Check sheet for the modelled part. Datum: model origin and axes. Units: mm. Face numbers are marked on the shaded views. A direction names the side the tool comes from. Give positions to 0.01 mm unless a question says otherwise; leave off trailing zeros. Loops run counter-clockwise (first coordinate to the right, second up) from the corner with the lowest first, then second, coordinate; pieces in that order, holes last.
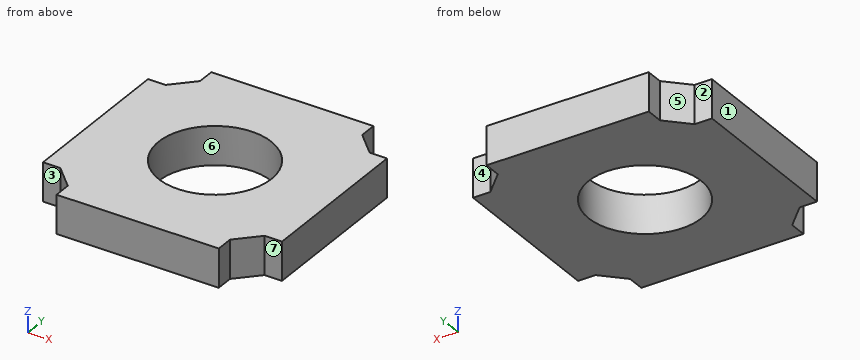
Autodesk Inventor part; units mm, degrees
ref_plane "YZ Plane" through (0, 0, 0) normal (1, 0, 0) x (0, 1, 0)
ref_plane "XZ Plane" through (0, 0, 0) normal (0, 1, 0) x (-1, 0, 0)
ref_plane "XY Plane" through (0, 0, 0) normal (0, 0, 1) x (1, 0, 0)
sketch "Sketch1" plane through (0, 0, 0) normal (0, 0, 1) x (1, 0, 0)
  line L0 (21.5871, 13.6345) -> (17.0871, 18.1345)
  line L1 (17.0871, 18.1345) -> (-16.7129, 18.1345)
  line L2 (-16.7129, 18.1345) -> (-21.2129, 13.6345)
  line L3 (-21.0966, 13.6345) -> (-21.0966, -20.1655)
  line L4 (21.4709, -20.1655) -> (21.4709, 13.6345)
  line L5 (21.4709, -20.1655) -> (17.0871, -24.4078)
  line L6 (-16.7129, -24.4078) -> (17.0871, -24.4078)
  line L7 (-16.7129, -24.4078) -> (-21.0966, -20.1655)
  line L8 (-24.7129, -28.1655) -> (-24.7129, 13.6345) construction
  line L9 (25.0871, -28.1655) -> (-24.7129, -28.1655) construction
  line L10 (25.0871, -28.1655) -> (25.0871, 13.6345) construction
  line L11 (17.0871, 21.6345) -> (-16.7129, 21.6345) construction
  line L12 (0.1871, -36.5255) -> (0.1871, 21.9945)
  line L13 (14.6206, -3.2655) -> (-14.2825, -3.2655) construction
  line L14 (-21.0552, -20.0655) -> (-16.6129, -24.5078)
  line L15 (-16.6129, -24.5078) -> (-16.6129, -28.1655)
  line L16 (-16.6129, -28.1655) -> (16.9871, -28.1655)
  line L17 (16.9871, -28.1655) -> (16.9871, -24.5078)
  line L18 (16.9871, -24.5078) -> (21.4295, -20.0655)
  line L19 (25.0871, -20.0655) -> (21.4295, -20.0655)
  line L20 (25.0871, 13.5345) -> (25.0871, -20.0655)
  line L21 (21.4295, 13.5345) -> (25.0871, 13.5345)
  line L22 (21.4295, 13.5345) -> (16.9871, 17.9768)
  line L23 (16.9871, 17.9768) -> (16.9871, 21.6345)
  line L24 (16.9871, 21.6345) -> (-16.6129, 21.6345)
  line L25 (-16.6129, 21.6345) -> (-16.6129, 17.9768)
  line L26 (-16.6129, 17.9768) -> (-21.0552, 13.5345)
  line L27 (-24.7129, 13.5345) -> (-21.0552, 13.5345)
  line L28 (-24.7129, -20.0655) -> (-24.7129, 13.5345)
  line L29 (-21.0552, -20.0655) -> (-24.7129, -20.0655)
  circle A0 centre (0.1871, -3.2655) radius 11.75
  point P0 (14.2, -44.8454)
  point P1 (11.9334, -2.9712)
  point P2 (-1.4501, -14.9009)
  point P3 (-5.6, -13.4915)
  point P4 (-9.0465, 4.0011)
  point P5 (-6.23, 6.5774)
  point P6 (11.3484, 0.4071)
  point P7 (16.9871, 19.8057)
  dimension "d48" = 23.5
extrude "Extrusion1" add sketch "Sketch1" along normal blind 8 contours L23 L22 L21 L4 L19 L18 L6 L12 A0 L1 | L1 L12 L24 L23 | L12 A0 L6 L14 L29 L3 L27 L26 L25 L1 | L1 L25 L24 L12 | L21 L20 L19 L4 | L12 L16 L15 L14 L6 | L6 L18 L17 L16 L12 | L3 L29 L28 L27
sketch "Skizze3" plane through (0, 0, 8) normal (0, 0, 1) x (1, 0, 0)
  circle A0 centre (0.1871, -3.2655) radius 11.75 construction
  line L0 (-21.0552, -20.0655) -> (-16.6129, -24.5078)
  line L1 (-16.6129, -24.5078) -> (-16.6129, -28.1655)
  line L2 (-16.6129, -28.1655) -> (16.9871, -28.1655) construction
  line L3 (16.9871, -28.1655) -> (16.9871, -24.5078)
  line L4 (16.9871, -24.5078) -> (21.4295, -20.0655)
  line L5 (21.4295, -20.0655) -> (25.0871, -20.0655)
  line L6 (25.0871, -20.0655) -> (25.0871, 13.5345) construction
  line L7 (25.0871, 13.5345) -> (21.4295, 13.5345)
  line L8 (21.4295, 13.5345) -> (16.9871, 17.9768)
  line L9 (16.9871, 17.9768) -> (16.9871, 21.6345)
  line L10 (16.9871, 21.6345) -> (-16.6129, 21.6345) construction
  line L11 (-16.6129, 21.6345) -> (-16.6129, 17.9768)
  line L12 (-16.6129, 17.9768) -> (-21.0552, 13.5345)
  line L13 (-21.0552, 13.5345) -> (-24.7129, 13.5345)
  line L14 (-24.7129, 13.5345) -> (-24.7129, -20.0655) construction
  line L15 (-24.7129, -20.0655) -> (-21.0552, -20.0655)
  line L16 (-16.7129, 21.7345) -> (17.0871, 21.7345) construction
  line L17 (17.0871, 21.7345) -> (17.0871, 18.0183)
  line L18 (17.0871, 18.0183) -> (21.4709, 13.6345)
  line L19 (21.4709, 13.6345) -> (25.1871, 13.6345)
  line L20 (25.1871, 13.6345) -> (25.1871, -20.1655) construction
  line L21 (25.1871, -20.1655) -> (21.4709, -20.1655)
  line L22 (21.4709, -20.1655) -> (17.0871, -24.5493)
  line L23 (17.0871, -24.5493) -> (17.0871, -28.2655)
  line L24 (17.0871, -28.2655) -> (-16.7129, -28.2655) construction
  line L25 (-16.7129, -28.2655) -> (-16.7129, -24.5493)
  line L26 (-16.7129, -24.5493) -> (-21.0966, -20.1655)
  line L27 (-21.0966, -20.1655) -> (-24.8129, -20.1655)
  line L28 (-24.8129, -20.1655) -> (-24.8129, 13.6345) construction
  line L29 (-24.8129, 13.6345) -> (-21.0966, 13.6345)
  line L30 (-21.0966, 13.6345) -> (-16.7129, 18.0183)
  line L31 (-16.7129, 18.0183) -> (-16.7129, 21.7345)
  line L32 (-21.0552, 13.5345) -> (-24.7129, 13.5345)
  line L33 (-24.7129, 13.5345) -> (-24.7129, 13.6345)
  line L34 (-16.6129, 21.6345) -> (-16.7129, 21.6345)
  line L35 (16.9871, 21.6345) -> (17.0871, 21.6345)
  line L36 (25.0871, 13.5345) -> (25.0871, 13.6345)
  line L37 (25.0871, -20.0655) -> (25.0871, -20.1655)
  line L38 (-16.6129, -28.1655) -> (16.9871, -28.1655)
  line L39 (16.9871, -28.1655) -> (17.0871, -28.1655)
  line L40 (-16.6129, -28.1655) -> (-16.7129, -28.1655)
  line L41 (-24.7129, -20.0655) -> (-24.7129, -20.1655)
  point P0 (0, 0)
  dimension "d52" = 0.1
extrude "IM_offset" add sketch "Skizze3" against normal up to surface (8 mm away)
properties part number "20_Cube_Insert_Holder-okular+flashlight_v3"
(1) Release check for a two-part mould opening along X. For the marked faces 5, 6 and 7 record: pulls with the +X half, pulls with the -X half, needs draft (parallel to the pull), parting line crosses it, or undercut.
(2) Section check B-B on x = 7.5. Record the boundary of the cut face in (y, z).
(3) Gauge pin test, flat ends, axial feed: pin 1 Ø3 at (x, z) = (23.5, 5.5) entering from -Y; pin 2 Ø1.8 at (y, z) = (-27, 5) entering from -X; pin 3 Ø1.8 at (x, z) = (22.5, 4) entering from +Y; pin 4 Ø1.5 at (y, z) = (-20.5, 5) entering from -X. Record the tip position at first contact, or that the pin passes through.
(4) Material ranges on line 1 (X direction, y = -8, z = 4.5); line 2 (X direction, y = -11.5, z = 6.5); line 3 (Y direction, x = -1, z = 5.25), recorded low to high.
(5) Section check C-C on z = 7. Record the boundary of the cut face in (x, y), plus the area to 3 significant figures.
(6) Section check A-A on y = 7.5. Record the boundary of the cut face in (x, z).
(7) Access from +Z, -Z, +X, -X, +Y, -Y to the whole of each face (thin tool, end or side, straight path). Record for the marked faces 1, 2, 3 and 4.
(8) Section check D-D on x = 19. Record the boundary of the cut face in (y, z).
Computed values:
1. face 5: pulls with the -X half
1. face 6: undercut
1. face 7: needs draft
2. outline: (-28.17, 0) - (-12.46, 0) - (-12.46, 8) - (-28.17, 8) - close; (5.93, 0) - (21.63, 0) - (21.63, 8) - (5.93, 8) - close
3. pin 1: stops at y = -20.17
3. pin 2: stops at x = -16.71
3. pin 3: stops at y = 13.63
3. pin 4: stops at x = -24.71
4. line 1: x = -24.71 to -10.57, 10.94 to 25.09
4. line 2: x = -24.71 to -8.19, 8.57 to 25.09
4. line 3: y = -28.17 to -14.96, 8.42 to 21.63
5. outline: (-24.71, -20.17) - (-21.1, -20.17) - (-16.71, -24.55) - (-16.71, -28.17) - (17.09, -28.17) - (17.09, -24.55) - (21.47, -20.17) - (25.09, -20.17) - (25.09, 13.63) - (21.47, 13.63) - (17.09, 18.02) - (17.09, 21.63) - (-16.71, 21.63) - (-16.71, 18.02) - (-21.1, 13.63) - (-24.71, 13.63) - close; hole circle Ø23.5 at (0.19, -3.27)
5. area: 1,830 mm2
6. outline: (-24.71, 0) - (-4.52, 0) - (-4.52, 8) - (-24.71, 8) - close; (4.9, 0) - (25.09, 0) - (25.09, 8) - (4.9, 8) - close
7. face 1: +Z, -Z, -X, +Y, -Y
7. face 2: +Z, -Z, -X, +Y
7. face 3: +Z, -Z, -X, -Y
7. face 4: +Z, -Z, +X, +Y
8. outline: (-22.64, 0) - (16.11, 0) - (16.11, 8) - (-22.64, 8) - close
